Verification items for the finished model (mm, model axes). A direction names the side the tool comes from. Coordinates: 2 decimals unless noted, no trailing zeros. Write each loop counter-clockwise with the first axis right and the second up, starting at its lowest first coordinate (ties: lowest second). Pieces come first, ordered by that corner, then holes.
```python
from build123d import *

# Parameters (mm, degrees)
F1_DEPTH = 63.5
F2_DEPTH = 25.4
F3_DEPTH = 7.9375
F4_W     = 25.4
F4_H     = 28.5877
F4_H_2   = 28.575
F4_H_3   = 20.5653703187
F6_R     = 3
F7_R     = 5.08


with BuildPart() as f1:
    # F0 (on Front) → F1 (new body, symmetric)
    with BuildSketch(Plane.XZ):
        Polygon((29.2099986579, 9.525), (-41.275, 9.525), (-41.275, -9.525), (41.275, -9.525), (41.275, 9.525), align=None)
    extrude(amount=F1_DEPTH, both=True)

    # F0 (on Front) → F2 (join, symmetric)
    with BuildSketch(Plane.XZ):
        with BuildLine():
            Line((29.2099986579, 27.0002), (29.2099986579, 9.525))
            Line((29.2099986579, 9.525), (41.275, 9.525))
            Line((41.275, 9.525), (41.275, 27.0002))
            ThreePointArc((41.275, 27.0002), (45.9246798487, 38.2255201513), (57.15, 42.8752))
            Line((57.15, 42.8752), (75.3208244484, 42.8752))
            Line((75.3208244484, 42.8752), (75.3208244484, 54.9402013421))
            Line((75.3208244484, 54.9402013421), (57.15, 54.9402013421))
            ThreePointArc((57.15, 54.9402013421), (37.3934355846, 46.7567644154), (29.2099986579, 27.0002))
        make_face()
        Polygon((75.3208244484, 57.1627), (75.3208244484, 54.9402013421), (75.3208244484, 42.8752), (75.3208244484, 28.5877), (126.1208244484, 28.5877), (126.1208244484, 57.1627), align=None)
    extrude(amount=F2_DEPTH, both=True)

    # F0 (on Front) → F3 (join, symmetric)
    with BuildSketch(Plane.XZ):
        with BuildLine():
            add(Edge.make_bspline(
                [(-41.275, 9.525), (-41.1590449512, 44.640161097), (4.4794571586, 56.3350282609), (57.15, 54.9402013421)],
                knots=[0, 0, 0, 0, 108.3975144454, 108.3975144454, 108.3975144454, 108.3975144454], degree=3))
            Line((-41.275, 9.525), (29.2099986579, 9.525))
            Line((29.2099986579, 9.525), (29.2099986579, 27.0002))
            ThreePointArc((29.2099986579, 27.0002), (37.3934355846, 46.7567644154), (57.15, 54.9402013421))
        make_face()
    extrude(amount=F3_DEPTH, both=True)

    # F4 (on face) → F5 (revolve)
    with BuildSketch(Plane.XZ.offset(25.4)):
        with Locations((113.4208244484, 14.29385)):
            Rectangle(F4_W, F4_H)
        with Locations((113.4208244484, 42.8752)):
            Rectangle(F4_W, F4_H_2)
        with Locations((113.4208244484, 67.4453851593)):
            Rectangle(F4_W, F4_H_3)
    revolve(axis=Axis((126.1208244484, 0, 42.8752), (0, 0, -1)))

    # F6
    f6_edges = [f1.edges().sort_by_distance(p)[0] for p in [
        (-41.275, 63.5, 0),
        (41.275, 63.5, 0),
        (-41.275, -63.5, 0),
    ]]
    fillet(f6_edges, radius=F6_R)

    # F7
    f7_edges = [f1.edges().sort_by_distance(p)[0] for p in [
        (37.393436, 25.4, 46.756764),
    ]]
    fillet(f7_edges, radius=F7_R)


solid = f1.part
```
1. Sectioned sample at B-B, the plane y = 17. Record the boundary of the cut face in (x, z) (3 decimals), and give its area (3 significant figures).
2. Sectioned sample at D-D, the plane z = 34. Give the number of separate pieces and of enclosed holes in the cut face, and give its area (3 significant figures).
3. Sectioned sample at C-C, the plane x = 72. Record the boundary of the cut face in (y, z), and give its area (3 significant figures).
4. Draft check along Y on faces 5 (the cylindrical face through (30.738, 23.951, 18.14)), 6 (the cylindrical face through (150.917, 5.506, 39.408)), 7 (the cylindrical face through (161.733, 4.701, 38.32)), 8 (the flat face through (85, 0, 57.163)). Enter one of: pulls with the +Y half, pulls with the -Y half, needs draft (parallel to the pull), parting line crosses it, or undercut.
5. Tool access check on faces 1 (the flat face through (41.275, -2, 4)), 2 (the flat face through (116, 0, 28.588)), 3 (the flat face through (116, 0, 57.163)), 4 (the cylindrical face through (37.61, 14.04, 46.97)). Record the directions out of +Z, -Z, +X, -X, +Y, -Y that give a thin tool (end or side, any length) a straight path to the whole face; none if there is none.
6. Sectioned sample at A-A, the plane x = 138.5. Record the boundary of the cut face in (y, z), and give its area (3 significant figures).
7. Gauge pin test, flat ends, axial feed: P1, Ø9, axis at x = 67, y = -2, coming from the +Z side; P2, Ø6, axis at y = 13, z = 16.5, coming from the -X side; P3, Ø12, axis at y = 4, z = 62, coming from the -X side. Record the tip position at first contact, or that the pin passes through.
8. Material ranges on L1, parallel to X at y = 20, z = 8 (3 decimals); L2, parallel to X at y = 0, z = 22 (3 decimals); L3, parallel to Z at x = -14.5, y = 29 (3 decimals), recorded low to high.
Outcome:
1. outline: (-41.275, -9.525) - (41.275, -9.525) - (41.275, 27) arc R15.875 cw to (57.15, 42.875) - (75.321, 42.875) - (75.321, 28.588) - (94.477, 28.588) - (94.477, 0) - (107.249, 0) - (107.249, 28.588) - (126.121, 28.588) - (126.121, 57.163) - (107.249, 57.163) - (107.249, 77.728) - (94.477, 77.728) - (94.477, 57.163) - (75.321, 57.163) - (75.321, 54.94) - (57.15, 54.94) arc R27.94 ccw to (29.21, 27) - (29.21, 9.525) - (-41.275, 9.525) - close; (144.993, 0) - (157.764, 0) - (157.764, 77.728) - (144.993, 77.728) - close
1. area: 5,490 mm2
2. separate pieces: 2
2. enclosed holes: 1
2. area: 5,580 mm2
3. outline: (-25.4, 42.88) - (25.4, 42.88) - (25.4, 49.86) arc R5.08 ccw to (20.32, 54.94) - (-25.4, 54.94) - close
3. area: 607 mm2
4. face 5: pulls with the +Y half
4. face 6: undercut
4. face 7: parting line crosses it
4. face 8: needs draft
5. face 1: -Z, +Y, -Y
5. face 2: -Z
5. face 3: +Z
5. face 4: +Z, -X, +Y
6. outline: (-33.72, 0) - (-22.18, 0) - (-22.18, 77.73) - (-33.72, 77.73) - close; (22.18, 0) - (33.72, 0) - (33.72, 77.73) - (22.18, 77.73) - close
6. area: 1,790 mm2
7. P1: stops at z = 54.94
7. P2: stops at x = 29.21
7. P3: stops at x = 75.32
8. L1: x = -41.275 to 41.275, 96.283 to 110.463, 141.778 to 155.959
8. L2: x = -39.028 to 41.275, 90.2 to 100.721, 151.521 to 162.042
8. L3: z = -9.525 to 9.525
